```python
from build123d import *

# Parameters (mm, degrees)
SKETCH1_R      = 3.175
EXTRUDE1_DEPTH = 2.9464
SKETCH2_R      = 1.4224
EXTRUDE2_DEPTH = 3.9464
CHAMFER1_SIZE  = 1.4224
CHAMFER1_SIZE2 = 0.995975202


with BuildPart() as part:
    # Sketch1 → Extrude1 (new body)
    with BuildSketch(Plane.XY):
        Circle(SKETCH1_R)
    extrude(amount=EXTRUDE1_DEPTH)

    # Sketch2 → Extrude2 (cut, through all)
    with BuildSketch(Plane.XY.offset(2.9464)):
        Circle(SKETCH2_R)
    extrude(amount=-EXTRUDE2_DEPTH, mode=Mode.SUBTRACT)

    # Chamfer1
    chamfer1_edges = [part.edges().sort_by_distance(p)[0] for p in [
        (-3.175, 0, 2.9464),
    ]]
    chamfer1_side = [part.faces().sort_by_distance(p)[0] for p in [
        (-3.175, 0, 1.4732),
    ]]
    chamfer(chamfer1_edges, length=CHAMFER1_SIZE, length2=CHAMFER1_SIZE2, reference=chamfer1_side[0])


solid = part.part
```
Geometry: final body of the model. Coordinates: model frame, mm. Round coordinates to 2 decimals unless told otherwise and drop trailing zeros. Write each loop counter-clockwise with the first axis right and the second up, starting at its lowest first coordinate (ties: lowest second). Pieces come first, ordered by that corner, then holes.
Item 1: Material intervals for L1, parallel to Y at x = 0, z = 0.8 (3 decimals); L2, parallel to X at y = 0.75, z = 2.1; L3, parallel to Y at x = 0, z = 1.95, sorted ascending.
Item 2: Mould query, pull axis X, two halves, no side actions, for faces 1 (the face through (-0.69, -3.1, 0.75)), 2 (the face through (-0.31, -1.39, 1.49)), 3 (the face through (1.4, 0.8, 0)). Classes: +X half, -X half, draft (parallel to the pull), parting line (faces both ways), or undercut.
Item 3: Section query A-A (y = 0). Return loops of the section in (x, z) (3 decimals), plus the area to 3 significant figures.
Item 4: Section query D-D (z = 2.15). Return loops of the section in (x, y).
Item 5: Section query C-C (z = 1.3). Return loops of the section in (x, y) (3 decimals).
Item 6: Pin query (flat end, axial travel): P1, Ø1.7, axis at x = 0, y = 0, coming from the +Z side. Return the tip coordinate at first contact, or that it passes through.
Completed:
1. L1: y = -3.175 to -1.422, 1.422 to 3.175
1. L2: x = -2.67 to -1.21, 1.21 to 2.67
1. L3: y = -2.88 to -1.42, 1.42 to 2.88
2. face 1: parting line
2. face 2: undercut
2. face 3: draft
3. outline: (-3.175, 0) - (-1.422, 0) - (-1.422, 2.946) - (-2.179, 2.946) - (-3.175, 1.524) - close; (1.422, 0) - (3.175, 0) - (3.175, 1.524) - (2.179, 2.946) - (1.422, 2.946) - close
3. area: 8.91 mm2
4. outline: circle Ø5.47 at (0, 0); hole circle Ø2.84 at (0, 0)
5. outline: circle Ø6.35 at (0, 0); hole circle Ø2.845 at (0, 0)
6. P1: passes through
